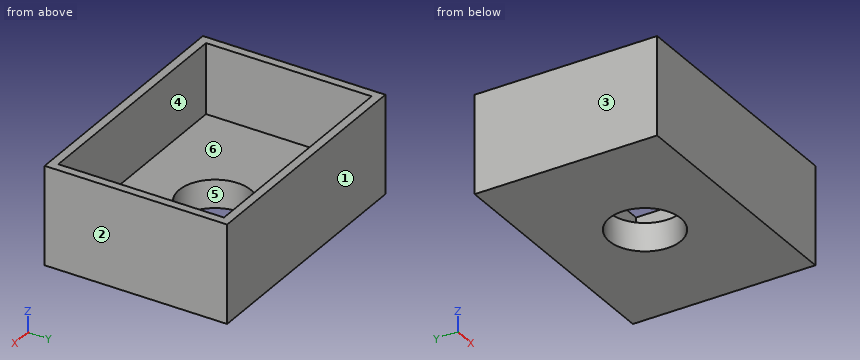
from build123d import *

# Parameters (mm, degrees)
F0_W     = 90
F0_H     = 65
F1_DEPTH = 10
F2_R     = 12.75
F3_DEPTH = 10
F4_W     = 90
F4_H     = 65
F4_W_2   = 84
F4_H_2   = 59
F5_DEPTH = 25


with BuildPart() as f1:
    # F0 (on Top) → F1 (new body)
    with BuildSketch(Plane.XY):
        Rectangle(F0_W, F0_H)
    extrude(amount=F1_DEPTH)

    # F2 (on face) → F3 (cut)
    with BuildSketch(Plane.XY.offset(10)):
        Circle(F2_R)
    extrude(amount=-F3_DEPTH, mode=Mode.SUBTRACT)

    # F4 (on face) → F5 (join)
    with BuildSketch(Plane.XY.offset(10)):
        Rectangle(F4_W, F4_H)
        Rectangle(F4_W_2, F4_H_2, mode=Mode.SUBTRACT)
    extrude(amount=F5_DEPTH)


solid = f1.part
Here's how the part is built. I have some questions about the finished solid (model axes, mm). Face numbers are marked on the shaded views. A direction names the side the tool comes from. Round coordinates to 2 decimals unless told otherwise and drop trailing zeros. Order: outer loops, then holes, each group sorted by start corner. A loop starts at its lowest first (then second) coordinate and runs counter-clockwise, first axis right, second up. Notation, with made-up numbers: M -8.5,25.5 L 31.5,25.5 A18 ccw 31.5,59.5 Z; hole C 47.5,37.5 d4. An arc over 180 degrees is marked long. Return JSON: item names as keys, results as strings. Group by question number.
1. If we section it at D-D on x = -24.5: List the corners of the cut face in (y, z) for me, then the cut area to 3 significant figures.
2. If we section it at A-A on x = 0: List the corners of the cut face in (y, z) for me, then the cut area to 3 significant figures.
3. If we section it at C-C on y = 16: List the corners of the cut face in (x, z) for me, then the cut area to 3 significant figures.
4. Please list where these lines run through material, in increasing order: probe 1 along Y at (x, z) = (-29, 21); probe 2 along Y at (x, z) = (0, 5.5); probe 3 along X at (y, z) = (-17, 17.5).
5. On a 3-axis mill with a long thin cutter (end or side, diameter ignored), from which of +Z, -Z, +X, -X, +Y, -Y can I reach the whole of each face in a straight line? I mean the marked faces 5 and 6. Say none if no direction works.
6. If we mould it in two halves opening along X, with no side actions, what happens to the marked faces 1, 2, 3 and 4? For each: pulls with the +X half, pulls with the -X half, needs draft (parallel to the pull), parting line crosses it, or undercut.
7. If we section it at B-B on z = 17: List the corners of the cut face in (x, y) for me, then the cut area to 3 significant figures.
Reply:
{
 "1": {"outline": "M -32.5,0 L 32.5,0 L 32.5,35 L 29.5,35 L 29.5,10 L -29.5,10 L -29.5,35 L -32.5,35 Z", "area": "800 mm^2"},
 "2": {"outline": "M -32.5,0 L -12.75,0 L -12.75,10 L -29.5,10 L -29.5,35 L -32.5,35 Z; M 12.75,0 L 32.5,0 L 32.5,35 L 29.5,35 L 29.5,10 L 12.75,10 Z", "area": "545 mm^2"},
 "3": {"outline": "M -45,0 L 45,0 L 45,35 L 42,35 L 42,10 L -42,10 L -42,35 L -45,35 Z", "area": "1,050 mm^2"},
 "4": {"probe 1": "-32.5 to -29.5, 29.5 to 32.5", "probe 2": "-32.5 to -12.75, 12.75 to 32.5", "probe 3": "-45 to -42, 42 to 45"},
 "5": {"face 5": "+Z, -Z", "face 6": "+Z"},
 "6": {"face 1": "needs draft", "face 2": "pulls with the +X half", "face 3": "pulls with the -X half", "face 4": "undercut"},
 "7": {"outline": "M -45,-32.5 L 45,-32.5 L 45,32.5 L -45,32.5 Z; hole M -42,-29.5 L 42,-29.5 L 42,29.5 L -42,29.5 Z", "area": "894 mm^2"}
}
